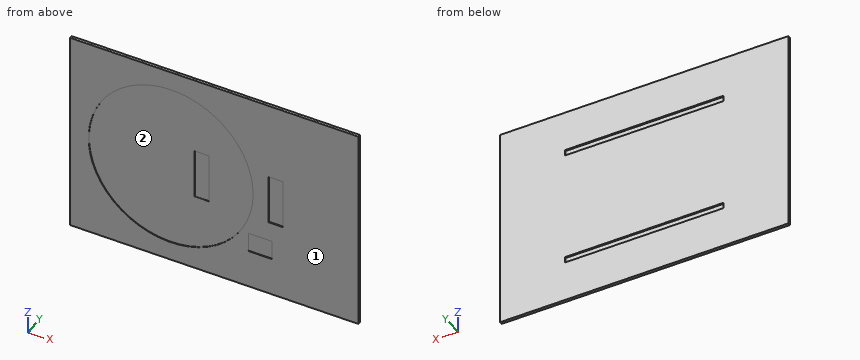
Autodesk Inventor part; units mm, degrees
ref_plane "YZ Plane" through (0, 0, 0) normal (1, 0, 0) x (0, 1, 0)
ref_plane "XZ Plane" through (0, 0, 0) normal (0, 1, 0) x (-1, 0, 0)
ref_plane "XY Plane" through (0, 0, 0) normal (0, 0, 1) x (1, 0, 0)
sketch "Sketch1" plane through (0, 0, 0) normal (0, 1, 0) x (-1, 0, 0)
  line L0 (500, -350) -> (-500, -350)
  line L1 (-500, -350) -> (-500, 350)
  line L2 (-500, 350) -> (500, 350)
  line L3 (500, 350) -> (500, -350)
  line L4 (500, -350) -> (-500, 350) construction
  line L5 (-500, -350) -> (500, 350) construction
  point P0 (0, 0)
  dimension "d0" = 1000
  dimension "d1" = 700
extrude "Extrusion1" add sketch "Sketch1" along normal blind 10
sketch "Sketch2" plane through (0, 10, 0) normal (0, 1, 0) x (1, 0, 0)
  line L0 (-500, -350) -> (500, -350)
  line L1 (500, -350) -> (500, 350)
  line L2 (500, 350) -> (-500, 350)
  line L3 (-500, 350) -> (-500, -350)
  line L4 (-275, -210) -> (275, -210) construction
  line L5 (275, -210) -> (275, 210) construction
  line L6 (275, 210) -> (-275, 210) construction
  line L7 (-275, 210) -> (-275, -210) construction
  line L8 (-275, -210) -> (275, 210) construction
  line L9 (275, -210) -> (-275, 210) construction
  line L10 (-275, -210) -> (275, -210)
  line L11 (275, -210) -> (275, -190)
  line L12 (275, -190) -> (-275, -190)
  line L13 (-275, -190) -> (-275, -210)
  line L14 (-275, 210) -> (275, 210)
  line L15 (275, 210) -> (275, 190)
  line L16 (275, 190) -> (-275, 190)
  line L17 (-275, 190) -> (-275, 210)
  point P0 (0, 0)
  dimension "d4" = 550
  dimension "d5" = 420
  dimension "d6" = 20
  dimension "d7" = 20
extrude "Extrusion2" cut sketch "Sketch2" against normal blind 5 contours L13 L12 L11 L10 | L14 L15 L16 L17
sketch "Sketch3" plane through (0, 0, 0) normal (0, -1, 0) x (1, 0, 0)
  line L0 (-500, 350) -> (500, 350)
  line L1 (-500, -350) -> (-500, 350)
  line L2 (500, -350) -> (-500, -350)
  line L3 (500, 350) -> (500, -350)
  line L4 (500, -350) -> (-500, -350) construction
  line L5 (0, -350) -> (0, 350) construction
  line L6 (-500, -350) -> (-500, 350) construction
  line L7 (-500, 0) -> (500, 0) construction
  circle A0 centre (-150, 0) radius 285
  circle A1 centre (-150, 0) radius 325 construction
  line L8 (200.7977, -218.4266) -> (118.3977, -218.4266)
  line L9 (118.3977, -218.4266) -> (118.3977, -152.0266)
  line L10 (118.3977, -152.0266) -> (200.7977, -152.0266)
  line L11 (200.7977, -152.0266) -> (200.7977, -218.4266)
  line L12 (-18.9239, 85) -> (-68.9239, 85)
  line L13 (-68.9239, 85) -> (-68.9239, -85)
  line L14 (-68.9239, -85) -> (-18.9239, -85)
  line L15 (-18.9239, -85) -> (-18.9239, 85)
  line L16 (239.0761, 85) -> (189.0761, 85)
  line L17 (189.0761, 85) -> (189.0761, -85)
  line L18 (189.0761, -85) -> (239.0761, -85)
  line L19 (239.0761, -85) -> (239.0761, 85)
  circle A2 centre (-150, 0) radius 160 construction
  line L20 (200.7977, -152.0266) -> (118.3977, -218.4266) construction
  line L21 (118.3977, -152.0266) -> (200.7977, -218.4266) construction
  circle A3 centre (159.5977, -185.2266) radius 48 construction
  line L22 (239.0761, -85) -> (189.0761, 85) construction
  line L23 (239.0761, 85) -> (189.0761, -85) construction
  line L24 (-18.9239, -85) -> (-68.9239, 85) construction
  line L25 (-18.9239, 85) -> (-68.9239, -85) construction
  line L26 (214.0761, 0) -> (-43.9239, 0) construction
  point P0 (0, 0)
  point P1 (85.0761, 0)
  dimension "d10" = 570
  dimension "d11" = 650
  dimension "d12" = 82.4
  dimension "d13" = 66.4
  dimension "d14" = 50
  dimension "d15" = 170
  dimension "d16" = 50
  dimension "d17" = 170
  dimension "d18" = 320
  dimension "d19" = 350
  dimension "d20" = 96
  dimension "d21" = 258
extrude "Extrusion3" cut sketch "Sketch3" against normal blind 1 contours A0 | L8 L9 L10 L11
extrude "Extrusion4" cut sketch "Sketch3" against normal blind 2 contours L15 L14 L13 L12 | L19 L18 L17 L16
extrude "Extrusion5" cut sketch "Sketch3" against normal blind 0.1 contours A0 | L8 L9 L10 L11
extrude "Extrusion6" cut sketch "Sketch3" against normal blind 1 contours A0 | L8 L9 L10 L11
extrude "Extrusion7" cut sketch "Sketch3" against normal blind 2 contours A0 | L8 L9 L10 L11
extrude "Extrusion8" cut sketch "Sketch3" against normal blind 3 contours L15 L14 L13 L12 | L19 L18 L17 L16
properties part number "Base Plate" material "Acetal Resin, White"
For this review, take the finished solid that the model builds, in its own axes (mm). Face numbers are marked on the shaded views. Coordinates: 2 decimals unless noted, no trailing zeros. Write each loop counter-clockwise with the first axis right and the second up, starting at its lowest first coordinate (ties: lowest second). Pieces come first, ordered by that corner, then holes. Notation, with made-up numbers: (-9, 29.25) - (48, 29.25) arc R23 ccw to (48, 59.25) - close; hole circle Ø9 at (69, 7). An arc over 180 degrees is marked (long way). Put each result on its own line as item: value.
1. Add section C-C, the plane x = -150. Give the boundary of the cut face in (y, z), then the cut area to 3 significant figures.
Values found:
outline: (0, -350) - (10, -350) - (10, -210) - (5, -210) - (5, -190) - (10, -190) - (10, 190) - (5, 190) - (5, 210) - (10, 210) - (10, 350) - (0, 350) - (0, 285) - (2, 285) - (2, -285) - (0, -285) - close
area: 5,660 mm²
2. Add section A-A, the plane z = 0. Give the boundary of the cut face in (x, y).
Values found:
outline: (-500, 0) - (-435, 0) - (-435, 2) - (-68.92, 2) - (-68.92, 3) - (-18.92, 3) - (-18.92, 2) - (135, 2) - (135, 0) - (189.08, 0) - (189.08, 3) - (239.08, 3) - (239.08, 0) - (500, 0) - (500, 10) - (-500, 10) - close
3. For pin 1 (25 mm diameter, centred on x = 207, z = 6.5, fed in from -Y); pin 2 (6 mm diameter, centred on x = 90, z = 199.5, fed in from +Y), all flat-tipped, find the tip position at first contact; note any pin that passes through.
Values found:
pin 1: y = 3
pin 2: y = 5
4. Add section D-D, the plane z = -242. Give the boundary of the cut face in (x, y), then the cut area to 3 significant figures.
Values found:
outline: (-500, 0) - (-300.54, 0) - (-300.54, 2) - (0.54, 2) - (0.54, 0) - (500, 0) - (500, 10) - (-500, 10) - close
area: 9,400 mm²
5. Mouldability with a two-part tool opening along X and no side actions: class the marked faces 1 and 2 as released by +X, released by -X, zero draft, split by the parting line, or undercut.
Values found:
face 1: zero draft
face 2: undercut
6. Wall thickness on probe 1 along Z at (x, y) = (-237.5, 9); probe 2 along X at (y, z) = (0.5, 9); probe 3 along Y at (x, z) = (-173, -248): over which ranges is each line inside the solid? List them lowest first.
Values found:
probe 1: -350 to -210, -190 to 190, 210 to 350
probe 2: -500 to -434.86, 134.86 to 189.08, 239.08 to 500
probe 3: 2 to 10
7. Add section B-B, the plane y = 8. Give the boundary of the cut face in (x, z).
Values found:
outline: (-500, -350) - (500, -350) - (500, 350) - (-500, 350) - close; hole (-275, -210) - (275, -210) - (275, -190) - (-275, -190) - close; hole (-275, 190) - (275, 190) - (275, 210) - (-275, 210) - close
